from build123d import *

# Parameters (mm, degrees)
BOSS_EXTRUDE3_DEPTH  = 6.35
SKETCH6_R            = 3.429
CUT_EXTRUDE5_DEPTH   = 6.35
FILLET2_R            = 2.5
SKETCH7_R            = 3.43
CUT_EXTRUDE6_DEPTH   = 144.750797039
SKETCH10_W           = 42.1894
SKETCH10_H           = 42.1894
CUT_EXTRUDE8_DEPTH   = 144.750797039
CUT_EXTRUDE9_DEPTH   = 2
SKETCH12_W           = 25.550132031
SKETCH12_H           = 25.4
CUT_EXTRUDE10_DEPTH  = 2
FILLET3_R            = 5
FILLET3_OF_MIRROR1_R = 5
CHAMFER1_SIZE        = 4.1


with BuildPart() as part:
    # Sketch1 → Boss-Extrude3 (new body)
    with BuildSketch(Plane.XY):
        Polygon((126.019412193, 68.87), (68.0566, 68.87), (62.2146, 68.87), (54.299929099, 68.87), (54.299929099, -68.87), (62.2146, -68.87), (126.019412193, -68.87), align=None)
    extrude(amount=BOSS_EXTRUDE3_DEPTH)

    # Sketch6 → Cut-Extrude5 (cut)
    with BuildSketch(Plane(origin=(0, 0, 0), x_dir=(-1, 0, 0), z_dir=(0, 0, -1))):
        with Locations((-63.5, 12.7)):
            Circle(SKETCH6_R)
        with Locations((-114.3, 38.1)):
            Circle(SKETCH6_R)
        with Locations((-114.3, -38.1)):
            Circle(SKETCH6_R)
        with Locations((-63.5, -12.7)):
            Circle(SKETCH6_R)
    extrude(amount=-CUT_EXTRUDE5_DEPTH, mode=Mode.SUBTRACT)

    # Fillet2
    fillet2_edges = [part.edges().sort_by_distance(p)[0] for p in [
        (54.299929099, 68.87, 3.175),
        (54.299929099, 0, 6.35),
        (90.159670646, -68.87, 6.35),
        (126.019412193, 0, 6.35),
        (90.159670646, 68.87, 6.35),
        (126.019412193, 68.87, 3.175),
        (126.019412193, -68.87, 3.175),
        (54.299929099, -68.87, 3.175),
    ]]
    fillet(fillet2_edges, radius=FILLET2_R)

    # Sketch7 → Cut-Extrude6 (cut, through all)
    with BuildSketch(Plane.XY.offset(6.35)):
        with Locations((90.159670646, 0)):
            Circle(SKETCH7_R)
    extrude(amount=-CUT_EXTRUDE6_DEPTH, mode=Mode.SUBTRACT)

    # Sketch10 → Cut-Extrude8 (cut, through all)
    with BuildSketch(Plane.XY.offset(6.35)):
        with Locations((101.606785129, 0)):
            Rectangle(SKETCH10_W, SKETCH10_H)
    extrude(amount=-CUT_EXTRUDE8_DEPTH, mode=Mode.SUBTRACT)

    # Sketch11 → Cut-Extrude9 (cut)
    with BuildSketch(Plane.XY.offset(6.35)):
        Polygon((123.519412193, -3), (122.701485129, -3), (122.701485129, 3), (123.519412193, 3), (127.39852583, 3), (127.39852583, -3), align=None)
    extrude(amount=-CUT_EXTRUDE9_DEPTH, mode=Mode.SUBTRACT)

    # Sketch12 → Cut-Extrude10 (cut)
    with BuildSketch(Plane.XY.offset(6.35)):
        with Locations((89.249266016, -36.599999996)):
            Rectangle(SKETCH12_W, SKETCH12_H)
    cut_extrude10 = extrude(amount=-CUT_EXTRUDE10_DEPTH, mode=Mode.SUBTRACT)

    # Fillet3
    fillet3_edges = [part.edges().sort_by_distance(p)[0] for p in [
        (76.4742, -49.299999996, 5.35),
        (76.4742, -23.899999996, 5.35),
        (102.024332031, -23.899999996, 5.35),
        (102.024332031, -49.299999996, 5.35),
    ]]
    fillet(fillet3_edges, radius=FILLET3_R)

    # Mirror1: Cut-Extrude10 across plane
    add(cut_extrude10.mirror(Plane(origin=(0, 0, 0), x_dir=(0, 0, 1), z_dir=(0, -1, 0))), mode=Mode.SUBTRACT)

    # Fillet3 of Mirror1
    fillet3_of_mirror1_edges = [part.edges().sort_by_distance(p)[0] for p in [
        (76.4742, 49.299999996, 5.35),
        (76.4742, 23.899999996, 5.35),
        (102.024332031, 23.899999996, 5.35),
        (102.024332031, 49.299999996, 5.35),
    ]]
    fillet(fillet3_of_mirror1_edges, radius=FILLET3_OF_MIRROR1_R)

    # Chamfer1
    chamfer1_edges = [part.edges().sort_by_distance(p)[0] for p in [
        (122.701485129, 21.0947, 3.175),
        (122.701485129, -21.0947, 3.175),
        (80.512085129, -21.0947, 3.175),
        (80.512085129, 21.0947, 3.175),
    ]]
    chamfer(chamfer1_edges, length=CHAMFER1_SIZE)


solid = part.part
Can you work these out from the model? Positions are in its coordinate system, mm. A direction names the side the tool comes from. Round coordinates to 2 decimals unless told otherwise and drop trailing zeros. Loops run counter-clockwise (first coordinate to the right, second up) from the corner with the lowest first, then second, coordinate; pieces in that order, holes last. Notation, with made-up numbers: (-2, -40) - (45, -40) arc R11 ccw to (45, -19) - close; hole circle Ø11 at (27, 66.25). An arc over 180 degrees is marked (long way). Use CSV: the item, a comma, the result in double quotes. Start each with the question number.
1) We'd pull the mould along Y, two halves only. Please class faces 4 (the cylindrical face through (125.307, -68.118, 1.952)), 5 (the flat face through (101, -21.095, 3)), 6 (the flat face through (54.3, 1, 2)), 7 (the cylindrical face through (100.521, -47.874, 5.336)): released by +Y, released by -Y, zero draft, split by the parting line, or undercut.
2) If we section it at C-C on y = -38.1: Write out the boundary of the cut face in (x, z), plus the area to 3 significant figures.
3) For faces 1 (the flat face through (74, 1, 0)), 2 (the flat face through (120.623, -19.073, 3.219)), 3 (the flat face through (89, 36, 4.35)), which set-ups out of +Z, -Z, +X, -X, +Y, -Y let a thin tool reach every point of the face, with its end or its side?
4) If we section it at D-D on x = 90.5: Write out the boundary of the cut face in (y, z), plus the area to 3 significant figures.
5) Please list where these lines run through material, in increasing order: probe 1 along Y at (x, z) = (114.3, 4); probe 2 along Y at (x, z) = (63.5, 3.25); probe 3 along Y at (x, z) = (113.5, 2.5). Write a range as [from, to].
6) If we section it at A-A on x = 114.3: Write out the boundary of the cut face in (y, z).
7) If we section it at B-B on y = -12.7: Write out the boundary of the cut face in (x, z), plus the area to 3 significant figures.
8) For pin 1 Ø2 at (x, z) = (86.5, 5.5) entering from -Y; pin 2 Ø1.5 at (x, z) = (114.5, 4.5) entering from +Y; pin 3 Ø0.6 at (x, z) = (123.5, 5.5) entering from +Y; pin 4 Ø12.5 at (x, y) = (93.5, 38) entering from +Z, each with a flat end and sliding along its axis, tell me the tip position at first contact or that it passes through.
Geometry results:
1,face 4,"released by -Y"
1,face 5,"undercut"
1,face 6,"zero draft"
1,face 7,"undercut"
2,outline,"(54.3, 0) - (110.87, 0) - (110.87, 6.35) - (102.02, 6.35) - (102.02, 4.35) - (76.47, 4.35) - (76.47, 6.35) - (56.8, 6.35) arc R2.5 ccw to (54.3, 3.85) - close; (117.73, 0) - (126.02, 0) - (126.02, 3.85) arc R2.5 ccw to (123.52, 6.35) - (117.73, 6.35) - close"
2,area,"358 mm2"
3,face 1,"-Z, +X, -X, +Y, -Y"
3,face 2,"+Z, -Z"
3,face 3,"+Z"
4,outline,"(-68.87, 0) - (-21.09, 0) - (-21.09, 6.35) - (-23.9, 6.35) - (-23.9, 4.35) - (-49.3, 4.35) - (-49.3, 6.35) - (-66.37, 6.35) arc R2.5 ccw to (-68.87, 3.85) - close; (21.09, 0) - (68.87, 0) - (68.87, 3.85) arc R2.5 ccw to (66.37, 6.35) - (49.3, 6.35) - (49.3, 4.35) - (23.9, 4.35) - (23.9, 6.35) - (21.09, 6.35) - close"
4,area,"502 mm2"
5,probe 1,"y = [-68.87, -41.53], [-34.67, -21.09], [21.09, 34.67], [41.53, 68.87]"
5,probe 2,"y = [-68.87, -16.13], [-9.27, 9.27], [16.13, 68.87]"
5,probe 3,"y = [-68.87, -41.43], [-34.77, -21.09], [21.09, 34.77], [41.43, 68.87]"
6,outline,"(-68.87, 0) - (-41.53, 0) - (-41.53, 6.35) - (-66.37, 6.35) arc R2.5 ccw to (-68.87, 3.85) - close; (-34.67, 0) - (-21.09, 0) - (-21.09, 6.35) - (-34.67, 6.35) - close; (21.09, 0) - (34.67, 0) - (34.67, 6.35) - (21.09, 6.35) - close; (41.53, 0) - (68.87, 0) - (68.87, 3.85) arc R2.5 ccw to (66.37, 6.35) - (41.53, 6.35) - close"
7,outline,"(54.3, 0) - (60.07, 0) - (60.07, 6.35) - (56.8, 6.35) arc R2.5 ccw to (54.3, 3.85) - close; (66.93, 0) - (80.51, 0) - (80.51, 6.35) - (66.93, 6.35) - close; (122.7, 0) - (126.02, 0) - (126.02, 3.85) arc R2.5 ccw to (123.52, 6.35) - (122.7, 6.35) - close"
7,area,"141 mm2"
8,pin 1,"stops at y = -68.78"
8,pin 2,"stops at y = 68.87"
8,pin 3,"stops at y = 68.47"
8,pin 4,"stops at z = 4.35"
